from build123d import *

# Parameters (mm, degrees)
BOSS_EXTRUDE1_DEPTH = 7
FILLET1_R           = 2
SKETCH3_R           = 1.5
SKETCH3_R_2         = 1.1
BOSS_EXTRUDE2_DEPTH = 4
SKETCH4_R           = 1.5
SKETCH4_R_2         = 0.640256745
SKETCH4_R_3         = 1.1
SKETCH4_W           = 1.5
SKETCH4_H           = 4.5
BOSS_EXTRUDE3_DEPTH = 4.5


with BuildPart() as part:
    # Sketch1 → Boss-Extrude1 (new body)
    with BuildSketch(Plane.XY):
        with BuildLine():
            Line((10, -9), (-10, -9))
            ThreePointArc((-10, -9), (-11.414213562, -8.414213562), (-12, -7))
            Line((-12, -7), (-12, 7))
            ThreePointArc((-12, 7), (-11.414213562, 8.414213562), (-10, 9))
            Line((-10, 9), (10, 9))
            ThreePointArc((10, 9), (11.414213562, 8.414213562), (12, 7))
            Line((12, 7), (12, -7))
            ThreePointArc((12, -7), (11.414213562, -8.414213562), (10, -9))
        make_face()
    extrude(amount=BOSS_EXTRUDE1_DEPTH)

    # Fillet1
    fillet1_edges = [part.edges().sort_by_distance(p)[0] for p in [
        (12, 0, 0),
        (11.414213562, -8.414213562, 0),
        (0, -9, 0),
        (-11.414213562, -8.414213562, 0),
        (11.414213562, -8.414213562, 7),
        (12, 0, 7),
        (11.414213562, 8.414213562, 7),
        (0, 9, 7),
        (-11.414213562, 8.414213562, 7),
        (-12, 0, 7),
        (-11.414213562, -8.414213562, 7),
        (-12, 0, 0),
        (0, -9, 7),
        (-11.414213562, 8.414213562, 0),
        (0, 9, 0),
        (11.414213562, 8.414213562, 0),
    ]]
    fillet(fillet1_edges, radius=FILLET1_R)

    # Sketch3 → Boss-Extrude2 (add)
    # profile 1 of 3: a face of its own
    with BuildSketch(Plane(origin=(12, 0, 0), x_dir=(0, 0, -1), z_dir=(1, 0, 0))):
        with Locations((-3.5, 7)):
            Circle(SKETCH3_R)
        with Locations((-3.5, 7)):
            Circle(SKETCH3_R_2, mode=Mode.SUBTRACT)
    # profile 2 of 3: a face of its own
    with BuildSketch(Plane(origin=(12, 0, 0), x_dir=(0, 0, -1), z_dir=(1, 0, 0))):
        with Locations((-3.5, 0.451158359)):
            Circle(SKETCH3_R)
        with Locations((-3.5, 0.451158359)):
            Circle(SKETCH3_R_2, mode=Mode.SUBTRACT)
    # profile 3 of 3: a face of its own
    with BuildSketch(Plane(origin=(12, 0, 0), x_dir=(0, 0, -1), z_dir=(1, 0, 0))):
        with Locations((-3.5, -6.097683282)):
            Circle(SKETCH3_R)
        with Locations(Location((-3.5, -6.097683282, 0), (0, 0, 235.113626632))):
            Circle(SKETCH3_R_2, mode=Mode.SUBTRACT)
    extrude(amount=BOSS_EXTRUDE2_DEPTH)

    # Sketch4 → Boss-Extrude3 (add)
    # profile 1 of 3: a face of its own
    with BuildSketch(Plane.ZY.offset(12)):
        with Locations((3.5, -0.844007622)):
            Circle(SKETCH4_R)
        with Locations((3.5, -0.844007622)):
            Circle(SKETCH4_R_2, mode=Mode.SUBTRACT)
    # profile 2 of 3: a face of its own
    with BuildSketch(Plane.ZY.offset(12)):
        with Locations((3.5, -5.244007622)):
            Circle(SKETCH4_R)
        with Locations((3.5, -5.244007622)):
            Circle(SKETCH4_R_3, mode=Mode.SUBTRACT)
    # profile 3 of 3: a face of its own
    with BuildSketch(Plane.ZY.offset(12)):
        with Locations((3.5, 5.420795306)):
            Rectangle(SKETCH4_W, SKETCH4_H)
    extrude(amount=BOSS_EXTRUDE3_DEPTH)


solid = part.part
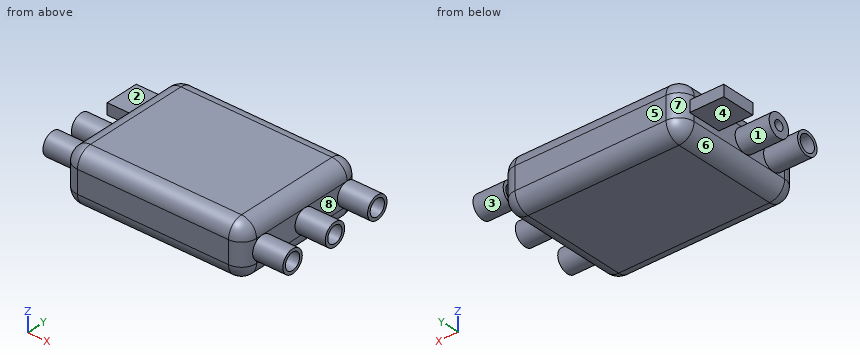
Work out the finished part from the listing and answer in its coordinate system (mm). Face numbers are marked on the shaded views. A direction names the side the tool comes from. Round coordinates to 2 decimals unless told otherwise and drop trailing zeros. Write each loop counter-clockwise with the first axis right and the second up, starting at its lowest first coordinate (ties: lowest second). Pieces come first, ordered by that corner, then holes. Notation, with made-up numbers: (-10, 56.5) -> (2, 56.5) arc R27 cw to (2, 84.5) -> close; hole circle Ø7 at (-10.75, 65). An arc over 180 degrees is marked (long way). Write each question's results on one line, items separated by ' | '.
Item 1: Find the intervals of material crossed by line 1 along Y through (x, z) = (13.1, 3.5); line 2 along Y through (x, z) = (-13.05, 3.5); line 3 along Y through (x, z) = (15.5, 2.75), in increasing order. Write a range as [from, to].
Result set:
line 1: [-7.6, -7.2], [-5, -4.6], [-1.05, -0.65], [1.55, 1.95], [5.5, 5.9], [8.1, 8.5] | line 2: [-6.74, -6.34], [-4.14, -3.74], [-2.34, -1.48], [-0.2, 0.66], [3.17, 7.67] | line 3: [-7.4, -6.9], [-5.29, -4.8], [-0.85, -0.35], [1.26, 1.75], [5.7, 6.2], [7.8, 8.3]
Item 2: A cutting plane is placed at D-D, the plane z = 3.5. Count the separate pieces of the cut face and the enclosed holes in it, plus the area to 3 significant figures.
Result set:
separate pieces: 3 | enclosed holes: 0 | area: 470 mm^2
Item 3: A cutting plane is placed at A-A, the plane x = -14. Determine the outline of the cut face in (y, z), plus the area to 3 significant figures.
Result set:
outline: circle Ø3 at (-5.24, 3.5); circle Ø3 at (-0.84, 3.5); (3.17, 2.75) -> (7.67, 2.75) -> (7.67, 4.25) -> (3.17, 4.25) -> close; hole circle Ø2.2 at (-5.24, 3.5); hole circle Ø1.28 at (-0.84, 3.5) | area: 15.8 mm^2
Item 4: Flat-ended cylindrical pins translate along their axes: P1, Ø2, axis at x = -14.5, y = 4.5, coming from the -Z side; P2, Ø3, axis at y = -6.5, z = 4.5, coming from the +X side; P3, Ø1.6, axis at x = -15.5, z = 4, coming from the -Y side; P4, Ø0.9, axis at y = 4.5, z = 3.5, coming from the +X side. Find the tip coordinate at first contact, or state that the pin passes through.
Result set:
P1: z = 2.75 | P2: x = 16 | P3: y = -6.74 | P4: x = 12
Item 5: A cutting plane is placed at B-B, the plane x = -6. Determine the outline of the cut face in (y, z).
Result set:
outline: (-9, 2) arc R2 ccw to (-7, 0) -> (7, 0) arc R2 ccw to (9, 2) -> (9, 5) arc R2 ccw to (7, 7) -> (-7, 7) arc R2 ccw to (-9, 5) -> close
Item 6: Which of the six approach directions +Z, -Z, +X, -X, +Y, -Y give full straight-line access (tool end or side, diameter ignored) to the marked faces 1, 2, 3 and 4?
Result set:
face 1: -X | face 2: +Z, -X, +Y | face 3: +X | face 4: -Z, -X, +Y
Item 7: The mould has two halves that part along X. Classify the marked faces 5, 6, 7 and 8: +X half, -X half, draft (parallel to the pull), parting line (faces both ways), or undercut.
Result set:
face 5: draft | face 6: -X half | face 7: undercut | face 8: +X half
Item 8: A cutting plane is placed at C-C, the plane z = 6.5. Determine the outline of the cut face in (x, y).
Result set:
outline: (-11.32, -7) arc R1.32 ccw to (-10, -8.32) -> (10, -8.32) arc R1.32 ccw to (11.32, -7) -> (11.32, 7) arc R1.32 ccw to (10, 8.32) -> (-10, 8.32) arc R1.32 ccw to (-11.32, 7) -> close
